Build history of the part. All positions in model axes, mm. A direction names the side the tool comes from. Round coordinates to 2 decimals unless told otherwise and drop trailing zeros. Order: outer loops, then holes, each group sorted by start corner. A loop starts at its lowest first (then second) coordinate and runs counter-clockwise, first axis right, second up. Notation, with made-up numbers: M 7,13.25 L 16,13.25 A32 ccw 16,42.25 Z; hole C 35,47 d6. An arc over 180 degrees is marked long. One line per item, written item: value. Start each with the question number.
Item 1: Tool access for faces 4 (the flat face through (11, 66, -8)), 5 (the cylindrical face through (7.056, 1.248, -4.437)), 6 (the flat face through (22.5, 104, -3)), 7 (the flat face through (39.2, 27.57, -8.01)), 8 (the flat face through (8, 60, -8)): list every direction of +Z, -Z, +X, -X, +Y, -Y with a clear straight run to the whole face (end or side of a thin tool).
Item 2: Band-saw the part on C-C, the plane y = 45.5. Write the cut outline in (x, z).
Item 3: Probe L1, parallel to Y at x = 38, z = -1; L2, parallel to Y at x = 18, z = -7.8; L3, parallel to Y at x = 32, z = 0.5. List the from-to ranges inside material, lowest first.
Item 4: Band-saw the part on A-A, the plane y = 98.5. Write the cut outline in (x, z).
Item 5: Pin check, flat tips, straight feed: pin 1 (5 mm diameter, centred on x = 38.5, z = -3.5, fed in from +Y); pin 2 (10 mm diameter, centred on x = 19, z = 3, fed in from -Y); pin 3 (1 mm diameter, centred on y = 61.5, z = 3.5, fed in from +X); pin 4 (1.6 mm diameter, centred on y = 92.5, z = -8.5, fed in from -X). Stop position of each tip, or through.
Item 6: Two-plate mould, pull along X, no slides. Class faces 1 (the cylindrical face through (41.03, 28.73, -8.01)), 2 (the flat face through (42, 47, -3)), 3 (the flat face through (14, 62, -4)): +X half, -X half, draft (parallel to the pull), parting line (faces both ways), or undercut.
```python
from build123d import *

# Parameters (mm, degrees)
EXTRUDE_1_DEPTH                 = 52
CUT_EXTRUDE_1_REACH             = 124.004
CUT_EXTRUDE_1_DIRECTION_2_DEPTH = 7
SKETCH_3_R                      = 1.5
CUT_EXTRUDE_2_DEPTH             = 123.167917229
SKETCH_5_R                      = 4
EXTRUDE_3_DEPTH                 = 8
FILLET_1_R                      = 5
CHAMFER_1_SIZE                  = 5
FILLET_2_R                      = 12.5
EXTRUDE_2_DEPTH                 = 9
CHAMFER_2_SIZE                  = 5
EXTRUDE_4_DEPTH                 = 9
EXTRUDE_4_DEPTH_BACK            = 2
CHAMFER_3_SIZE                  = 2
SKETCH_7_R                      = 1.6
EXTRUDE_5_DEPTH                 = 2


with BuildPart() as part:
    # 草图1 → 凸台-拉伸1 (new body)
    with BuildSketch(Plane(origin=(0, 0, 0), x_dir=(0, 0, -1), z_dir=(1, 0, 0))):
        Polygon((0, 0), (0, 58), (9, 58), (9, 110), (7, 110), (7, 60), (-2, 60), (-2, 0), align=None)
    extrude(amount=EXTRUDE_1_DEPTH)

    # 草图2 → 切除-拉伸1 (cut, up to next)
    with BuildSketch(Plane.XY.offset(-7), mode=Mode.PRIVATE) as cut_extrude_1_sk1:
        Polygon((24, 106), (49, 106), (49, 83), (24, 83), (24, 88.5), (14, 88.5), (14, 77), (41, 77), (41, 66), (31, 66), (31, 58), (17, 58), (17, 66), (4, 66), (4, 100.5), (24, 100.5), align=None)
    cut_extrude_1_tool1 = extrude(cut_extrude_1_sk1.sketch, amount=-CUT_EXTRUDE_1_REACH, mode=Mode.PRIVATE) & part.part
    add(cut_extrude_1_tool1.solids().sort_by_distance((25.692202, 84.595066, -7))[0], mode=Mode.SUBTRACT)

    # 草图2 → 切除-拉伸1 direction 2 (cut)
    with BuildSketch(Plane.XY.offset(-7)):
        Polygon((24, 106), (49, 106), (49, 83), (24, 83), (24, 88.5), (14, 88.5), (14, 77), (41, 77), (41, 66), (31, 66), (31, 58), (17, 58), (17, 66), (4, 66), (4, 100.5), (24, 100.5), align=None)
    extrude(amount=CUT_EXTRUDE_1_DIRECTION_2_DEPTH, mode=Mode.SUBTRACT)

    # 草图3 → 切除-拉伸2 (cut, through all)
    with BuildSketch(Plane.XY.offset(2)):
        with Locations((8, 105)):
            Circle(SKETCH_3_R)
        with Locations((18, 105)):
            Circle(SKETCH_3_R)
        with Locations((47, 76)):
            Circle(SKETCH_3_R)
        with BuildLine():
            Line((0, 60), (11.791303716, 60))
            ThreePointArc((11.791303716, 60), (9.662737441, 38.416613409), (0, 19))
            Line((0, 19), (0, 60))
        make_face()
        Polygon((42, 35), (42, 60), (52, 75), (52, 0), (22, 0), align=None)
    extrude(amount=-CUT_EXTRUDE_2_DEPTH, mode=Mode.SUBTRACT)

    # 草图5 → 凸台-拉伸3 (add)
    with BuildSketch(Plane(origin=(0, 0, 0), x_dir=(-1, 0, 0), z_dir=(0, 0, -1))):
        with Locations(Location((-12, 12, 0), (0, 0, 90))):
            Circle(SKETCH_5_R)
    extrude(amount=-EXTRUDE_3_DEPTH)

    # 圆角1
    fillet_1_edges = [part.edges().sort_by_distance(p)[0] for p in [
        (52, 75, -8),
        (0, 60, -8),
        (52, 110, -8),
        (0, 110, -8),
    ]]
    fillet(fillet_1_edges, radius=FILLET_1_R)

    # 倒角1
    chamfer_1_edges = [part.edges().sort_by_distance(p)[0] for p in [
        (14.395651858, 60, -7),
        (36.5, 60, -7),
    ]]
    chamfer(chamfer_1_edges, length=CHAMFER_1_SIZE)

    # 圆角2
    fillet_2_edges = [part.edges().sort_by_distance(p)[0] for p in [
        (22, 0, 1),
        (0, 0, 1),
        (0, 19, 1),
    ]]
    fillet(fillet_2_edges, radius=FILLET_2_R)

    # 草图4 → 凸台-拉伸2 (add)
    with BuildSketch(Plane.XY.offset(-7)):
        Polygon((24, 88.5), (24, 83), (49, 83), (49, 106), (24, 106), (24, 100.5), (22.5, 100.5), (22.5, 107.5), (50.5, 107.5), (50.5, 81.5), (45, 81.5), (42, 60), (40.485467906, 60), (43.485467906, 81.5), (22.5, 81.5), (22.5, 88.5), align=None)
    extrude(amount=EXTRUDE_2_DEPTH)

    # 倒角2
    chamfer_2_edges = [part.edges().sort_by_distance(p)[0] for p in [
        (14.462476533, 58, 0),
        (36.5, 58, 0),
    ]]
    chamfer(chamfer_2_edges, length=CHAMFER_2_SIZE)

    # 草图6 → 凸台-拉伸4 (add, two sides: drawn at the far end of the back side and taken through both)
    with BuildSketch(Plane(origin=(0, 0, 0), x_dir=(-1, 0, 0), z_dir=(0, 0, -1)).offset(-EXTRUDE_4_DEPTH_BACK)):
        with BuildLine():
            Line((-40.5, 60), (-42, 60))
            Line((-42, 60), (-42, 35))
            Line((-42, 35), (-25.599007583, 6.298263271))
            Line((-25.599007583, 6.298263271), (-22.133485774, 2.341459168))
            ThreePointArc((-22.133485774, 2.341459168), (-6.971383575, -0.362130478), (1.5, 12.5))
            Line((1.5, 12.5), (0, 12.5))
            ThreePointArc((0, 12.5), (-7.235227504, 1.162797057), (-20.565147291, 2.949952923))
            Line((-20.565147291, 2.949952923), (-24.572792271, 7.525733129))
            Line((-24.572792271, 7.525733129), (-40.5, 35.398346656))
            Line((-40.5, 35.398346656), (-40.5, 60))
        make_face()
    extrude(amount=EXTRUDE_4_DEPTH + EXTRUDE_4_DEPTH_BACK)

    # 倒角3
    chamfer_3_edges = [part.edges().sort_by_distance(p)[0] for p in [
        (12, 8, 2),
    ]]
    chamfer(chamfer_3_edges, length=CHAMFER_3_SIZE)

    # 草图7 → 凸台-拉伸5 (add)
    with BuildSketch(Plane(origin=(0, 0, -9), x_dir=(-1, 0, 0), z_dir=(0, 0, -1))):
        with BuildLine():
            Line((-41.58264013, 34.269620228), (-43.736486284, 33.038850997))
            ThreePointArc((-43.736486284, 33.038850997), (-45.038850997, 28.263513716), (-40.263513716, 26.961149003))
            Line((-40.263513716, 26.961149003), (-38.109667562, 28.191918233))
            Line((-38.109667562, 28.191918233), (-41.58264013, 34.269620228))
        make_face()
        with Locations(Location((-42, 30, 0), (0, 0, 90))):
            Circle(SKETCH_7_R, mode=Mode.SUBTRACT)
    extrude(amount=-EXTRUDE_5_DEPTH)


solid = part.part
```
Output:
1. face 4: +Z, -Z
1. face 5: -Z
1. face 6: +Z, -X, +Y
1. face 7: +Z, -Z, -Y
1. face 8: +Z, -Z, -X
2. outline: M 11.24,0 L 40.5,0 L 40.5,-9 L 42,-9 L 42,2 L 11.24,2 Z
3. L1: y = 28 to 31.02, 54 to 60, 81.5 to 83, 106 to 107.5
3. L2: y = -0.37 to 1.28, 77 to 88.5, 100.5 to 103.5, 106.5 to 110
3. L3: y = 17.5 to 60, 81.5 to 83, 106 to 107.5
4. outline: M 0,-9 L 4,-9 L 4,-7 L 0,-7 Z; M 49,-9 L 52,-9 L 52,-7 L 50.5,-7 L 50.5,2 L 49,2 Z
5. pin 1: stops at y = 107.5
5. pin 2: stops at y = -1.41
5. pin 3: passes through
5. pin 4: stops at x = 0
6. face 1: undercut
6. face 2: +X half
6. face 3: draft
